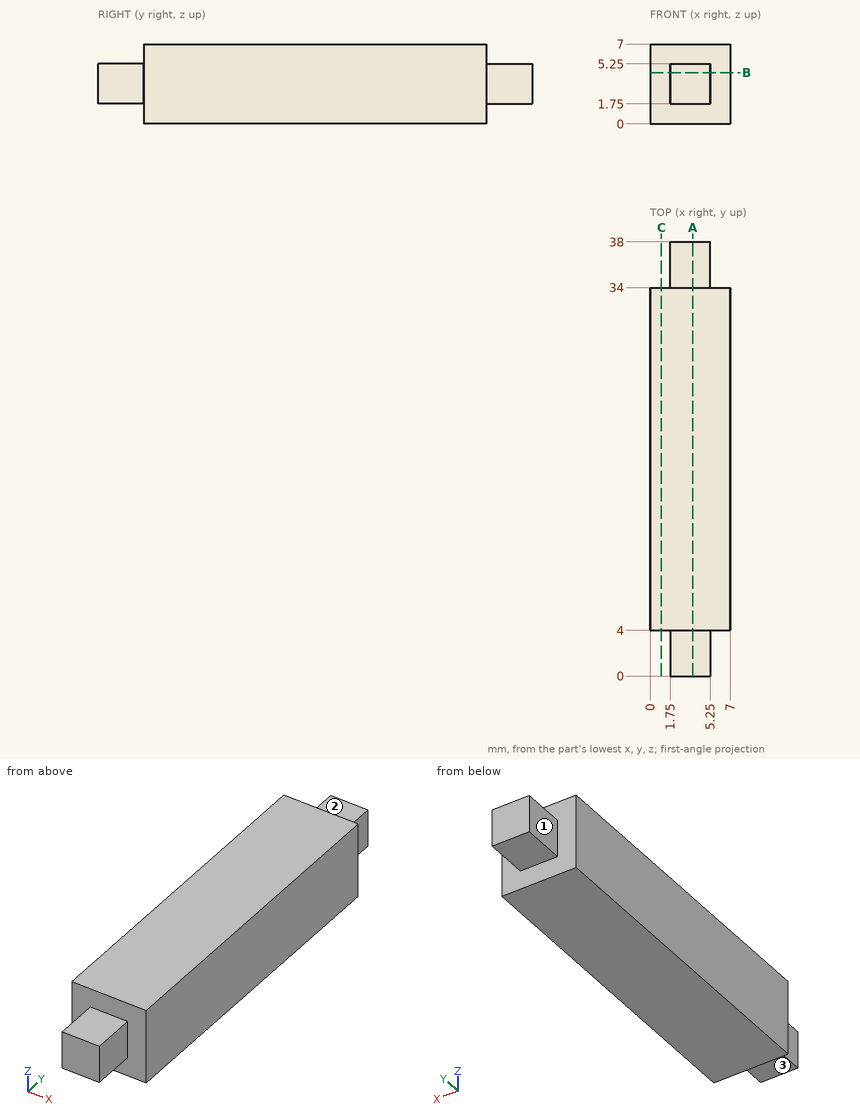
The drawing under review shows one solid part. Ordinate dimensions are in mm from its lowest x, y, z. A direction names the side the tool comes from. Round coordinates to 2 decimals unless told otherwise and drop trailing zeros. Loops run counter-clockwise (first coordinate to the right, second up) from the corner with the lowest first, then second, coordinate; pieces in that order, holes last. Notation, with made-up numbers: (62, -36) - (116, -36) arc R17 cw to (116, -13) - close; hole circle Ø7 at (5, -12.75). An arc over 180 degrees is marked (long way). One line per item, written item: value. Start each with the question number.
1) Consider section A-A on x = 3.75. Give the boundary of the cut face in (y, z).
2) For the marked faces 1, 2 and 3, list the 3-axis set-ups (+Z, -Z, +X, -X, +Y, -Y) from which the entire face can be reached by the end or side of a thin tool; tool diameter is ignored.
3) Consider section C-C on x = 1. Give the boundary of the cut face in (y, z), then the cut area to 3 significant figures.
4) Insertion check: pin 1 Ø4 at (y, z) = (36.5, 3) entering from -X; pin 2 Ø1 at (x, y) = (2.5, 1.5) entering from +Z; pin 3 Ø1 at (y, z) = (36.5, 4.5) entering from +X. Each pin has a flat end and moves straight along its axis. Give the tip position at first contact, or say it passes through.
5) To check wall thickness, follow L1, parallel to X at y = 3, z = 5; L2, parallel to Y at x = 5.5, z = 3.75. State the ranges of each line that lie inside material, in increasing order. Write a range as from..to.
6) Consider section B-B on z = 4.5. Give the boundary of the cut face in (x, y), then the cut area to 3 significant figures.
Reported:
1. outline: (0, 1.75) - (4, 1.75) - (4, 0) - (34, 0) - (34, 1.75) - (38, 1.75) - (38, 5.25) - (34, 5.25) - (34, 7) - (4, 7) - (4, 5.25) - (0, 5.25) - close
2. face 1: +Z, -Z, -X, +Y
2. face 2: +Z, +X, -X, +Y
2. face 3: -Z, +X, -X, -Y
3. outline: (4, 0) - (34, 0) - (34, 7) - (4, 7) - close
3. area: 210 mm^2
4. pin 1: stops at x = 1.75
4. pin 2: stops at z = 5.25
4. pin 3: stops at x = 5.25
5. L1: x = 1.75..5.25
5. L2: y = 4..34
6. outline: (0, 4) - (1.75, 4) - (1.75, 0) - (5.25, 0) - (5.25, 4) - (7, 4) - (7, 34) - (5.25, 34) - (5.25, 38) - (1.75, 38) - (1.75, 34) - (0, 34) - close
6. area: 238 mm^2
